Input: part model. Units: mm. Frame: model coordinates. A direction names the side the tool comes from. Coordinates: 2 decimals unless noted, no trailing zeros. Write each loop counter-clockwise with the first axis right and the second up, starting at its lowest first coordinate (ties: lowest second). Pieces come first, ordered by that corner, then holes.
1) Section query B-B (z = -6). Output: boundary loops of the cut face in (x, y).
2) Section query C-C (x = 6). Output: boundary loops of the cut face in (y, z).
3) Section query A-A (x = 0). Output: boundary loops of the cut face in (y, z), then the cut area to 3 significant figures.
4) Line query: L1, parallel to X at y = 1.5, z = -4; L2, parallel to Z at x = -3, y = 7; L3, parallel to Z at x = 12, y = 3.75. Output: solid intervals per line, ascending.
5) Set-up query: faces 5 (the cylindrical face through (14.485, 2.921, -1.064)), 6 (the flat face through (8, 4, -4)). Return all of +Z, -Z, +X, -X, +Y, -Y with unobstructed straight access to the full face (end or side cutting, diameter ignored); none if empty.
6) Section query D-D (z = 8.5). State how many separate pieces and enclosed holes the cut face has, then the cut area to 3 significant figures.
7) Pin query (flat end, axial travel): pin 1 Ø4 at (y, z) = (6.5, -8) entering from +X; pin 2 Ø4 at (x, z) = (-2, 2) entering from +Y; pin 3 Ø6 at (x, z) = (-6.5, -1) entering from -Y; pin 4 Ø1.9 at (y, z) = (6.5, -1.5) entering from +X. Return the tip coordinate at first contact, or that it passes through.
8) Draft query along Z for faces 1 (the flat face through (0, 5, -10)), 2 (the cylindrical face through (6.39, 0.99, -2.38)), 3 (the flat face through (0, 5, -8)), 4 (the flat face through (-8, 4, -4)). Return one class per face: pulls with the +Z half, pulls with the -Z half, needs draft (parallel to the pull), parting line crosses it, or undercut.
from build123d import *

# Parameters (mm, degrees)
SKETCH1_R               = 2.6
BOSS_EXTRUDE3_DEPTH     = 20
SKETCH2_W               = 16
SKETCH2_H               = 16
CUT_EXTRUDE1_DEPTH      = 18
CUT_EXTRUDE2_DEPTH      = 34.915335764
CUT_EXTRUDE2_DEPTH_BACK = 34.915335764
CUT_EXTRUDE3_DEPTH      = 22.802901488
CUT_EXTRUDE3_DEPTH_BACK = 22.802901488
SKETCH5_R               = 1.75
SKETCH7_R               = 2.5
SKETCH7_R_2             = 1.75
BOSS_EXTRUDE4_DEPTH     = 4
CUT_EXTRUDE6_START      = -6.310905
SKETCH7_5_R             = 2.5
SKETCH7_5_R_2           = 1.75
CUT_EXTRUDE6_DEPTH      = 2.310905
SKETCH9_R               = 2.4
BOSS_EXTRUDE5_DEPTH     = 3


with BuildPart() as part:
    # Sketch1 → Boss-Extrude3 (new body)
    with BuildSketch(Plane(origin=(0, 0, 0), x_dir=(1, 0, 0), z_dir=(0, 1, 0))):
        with BuildLine():
            Line((-7.5, 10), (7.5, 10))
            ThreePointArc((7.5, 10), (17.5, 0), (7.5, -10))
            Line((7.5, -10), (-7.5, -10))
            ThreePointArc((-7.5, -10), (-17.5, 0), (-7.5, 10))
        make_face()
        with Locations(Location((-3.81, 2.042862393, 0), (0, 0, 270))):
            Circle(SKETCH1_R, mode=Mode.SUBTRACT)
        with Locations(Location((3.81, 2.042862393, 0), (0, 0, 270))):
            Circle(SKETCH1_R, mode=Mode.SUBTRACT)
        with Locations(Location((0, -2.042862393, 0), (0, 0, 270))):
            Circle(SKETCH1_R, mode=Mode.SUBTRACT)
    extrude(amount=BOSS_EXTRUDE3_DEPTH)

    # Sketch2 → Cut-Extrude1 (cut)
    with BuildSketch(Plane(origin=(0, 20, 0), x_dir=(1, 0, 0), z_dir=(0, 1, 0))):
        Rectangle(SKETCH2_W, SKETCH2_H)
    extrude(amount=-CUT_EXTRUDE1_DEPTH, mode=Mode.SUBTRACT)

    # Sketch4 → Cut-Extrude2 (cut, two sides: drawn at the far end of the back side and taken through both)
    with BuildSketch(Plane(origin=(-8, 0, 0), x_dir=(0, 0, -1), z_dir=(1, 0, 0)).offset(-CUT_EXTRUDE2_DEPTH_BACK)):
        Polygon((-8, 2), (-5.710986159, 2), (8, 8.393537847), (8, 20), (-8, 20), align=None)
        Polygon((8, 20), (8, 8.393537847), (10, 9.326153163), (10, 20), align=None)
        Polygon((-10, 20), (-10, 0), (-5.710986159, 2), (-8, 2), (-8, 20), align=None)
    extrude(amount=CUT_EXTRUDE2_DEPTH + CUT_EXTRUDE2_DEPTH_BACK, mode=Mode.SUBTRACT)

    # Sketch5 → Cut-Extrude3 (cut, two sides: drawn at the far end of the back side and taken through both)
    with BuildSketch(Plane(origin=(0, 3.830222216, 1.786061952), x_dir=(1, 0, 0), z_dir=(0, 0.9063077870366478, 0.42261826174070405)).offset(-CUT_EXTRUDE3_DEPTH_BACK)):
        with Locations(Location((-12.75, 1.970701319, 0), (0, 0, 270))):
            Circle(SKETCH5_R)
        with Locations(Location((12.75, 1.970701319, 0), (0, 0, 270))):
            Circle(SKETCH5_R)
    extrude(amount=CUT_EXTRUDE3_DEPTH + CUT_EXTRUDE3_DEPTH_BACK, mode=Mode.SUBTRACT)

    # Sketch7 → Boss-Extrude4 (add)
    # profile 1 of 2: a face of its own
    with BuildSketch(Plane(origin=(0, 3.830222216, 1.786061952), x_dir=(1, 0, 0), z_dir=(0, 0.9063077870366478, 0.42261826174070405))):
        with Locations((-12.75, 1.970701319)):
            Circle(SKETCH7_R)
        with Locations(Location((-12.75, 1.970701319, 0), (0, 0, 270))):
            Circle(SKETCH7_R_2, mode=Mode.SUBTRACT)
    # profile 2 of 2: a face of its own
    with BuildSketch(Plane(origin=(0, 3.830222216, 1.786061952), x_dir=(1, 0, 0), z_dir=(0, 0.9063077870366478, 0.42261826174070405))):
        with Locations((12.75, 1.970701319)):
            Circle(SKETCH7_R)
        with Locations(Location((12.75, 1.970701319, 0), (0, 0, 270))):
            Circle(SKETCH7_R_2, mode=Mode.SUBTRACT)
    extrude(amount=-BOSS_EXTRUDE4_DEPTH)

    # Sketch7<5> → Cut-Extrude6 (cut)
    # profile 1 of 2: a face of its own
    with BuildSketch(Plane(origin=(0, 3.830222216, 1.786061952), x_dir=(1, 0, 0), z_dir=(0, 0.9063077870366478, 0.42261826174070405)).offset(CUT_EXTRUDE6_START)):
        with Locations((-12.75, 1.970701319)):
            Circle(SKETCH7_5_R)
        with Locations(Location((-12.75, 1.970701319, 0), (0, 0, 270))):
            Circle(SKETCH7_5_R_2, mode=Mode.SUBTRACT)
    # profile 2 of 2: a face of its own
    with BuildSketch(Plane(origin=(0, 3.830222216, 1.786061952), x_dir=(1, 0, 0), z_dir=(0, 0.9063077870366478, 0.42261826174070405)).offset(CUT_EXTRUDE6_START)):
        with Locations((12.75, 1.970701319)):
            Circle(SKETCH7_5_R)
        with Locations(Location((12.75, 1.970701319, 0), (0, 0, 270))):
            Circle(SKETCH7_5_R_2, mode=Mode.SUBTRACT)
    extrude(amount=CUT_EXTRUDE6_DEPTH, mode=Mode.SUBTRACT)

    # Sketch9 → Boss-Extrude5 (add)
    with BuildSketch(Plane(origin=(0, 3.830222216, 1.786061952), x_dir=(1, 0, 0), z_dir=(0, 0.9063077870366478, 0.4226182617407042))):
        with Locations(Location((-11, -4.330674704, 0), (0, 0, 90))):
            Circle(SKETCH9_R)
        with Locations(Location((11, -4.330674704, 0), (0, 0, 90))):
            Circle(SKETCH9_R)
    extrude(amount=BOSS_EXTRUDE5_DEPTH)


solid = part.part
Answer:
1. outline: (-15.5, 0) - (15.5, 0) - (15.5, 7.46) - (8, 7.46) - (8, 2) - (-8, 2) - (-8, 7.46) - (-15.5, 7.46) - close
2. outline: (0, -10) - (9.33, -10) - (8.39, -8) - (2, -8) - (2, -3.44) - (0, -3.44) - close; (0, -0.64) - (2, -0.64) - (2, 5.71) - (0, 10) - close
3. outline: (0, -10) - (9.33, -10) - (8.39, -8) - (2, -8) - (2, -0.56) - (0, -0.56) - close; (0, 4.64) - (2, 4.64) - (2, 5.71) - (0, 10) - close
3. area: 39.0 mm2
4. L1: x = -16.67 to -13.76, -11.74 to -5.52, -2.1 to 2.1, 5.52 to 11.74, 13.76 to 16.67
4. L2: z = -10 to -8
4. L3: z = -8.93 to -2.17, 1.32 to 1.96, 4.12 to 8.93
5. face 5: none
5. face 6: +Z, +Y
6. separate pieces: 3
6. enclosed holes: 0
6. area: 25.9 mm2
7. pin 1: stops at x = 15.5
7. pin 2: stops at y = 2
7. pin 3: stops at y = 0
7. pin 4: passes through
8. face 1: pulls with the -Z half
8. face 2: undercut
8. face 3: pulls with the +Z half
8. face 4: needs draft
